```python
from build123d import *

# Parameters (mm, degrees)
F1_DEPTH = 100
F2_T     = -12
F4_W     = 187.6861900091
F4_H     = 13.1353894249
F5_DEPTH = 200


with BuildPart() as f1:
    # F0 (on Right) → F1 (new body, symmetric)
    with BuildSketch(Plane.YZ):
        Polygon((-193.7253567732, -86.0714143496), (-193.7253567732, -126.0714143496), (156.2746432268, -126.0714143496), (156.2746432268, 123.9285856504), (76.2746432268, 123.9285856504), align=None)
    extrude(amount=F1_DEPTH, both=True)

    # F2
    f2_openings = [f1.faces().sort_by_distance(p)[0] for p in [
        (0, -58.725357, 18.928586),
    ]]
    offset(amount=F2_T, openings=f2_openings)

    # F4 (on face) → F5 (join)
    with BuildSketch(Plane.YZ.offset(100)):
        with Locations((59.6075579524, 6.5676947124)):
            Rectangle(F4_W, F4_H)
    extrude(amount=-F5_DEPTH)


solid = f1.part
```
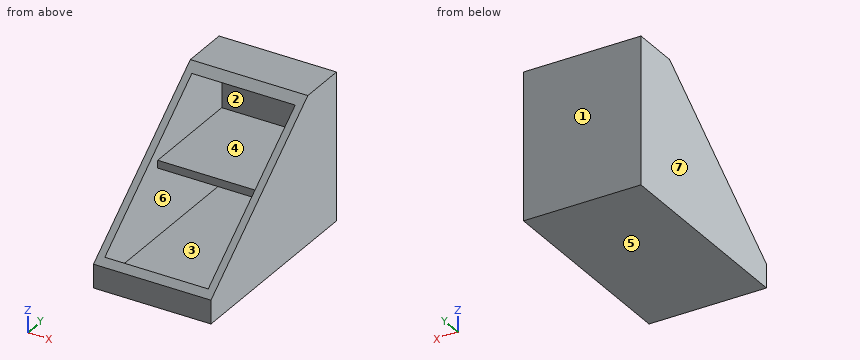
Work out the finished part from the listing and answer in its coordinate system (mm). Face numbers are marked on the shaded views. A direction names the side the tool comes from. Give positions to 0.01 mm unless a question says otherwise; leave off trailing zeros. Loops run counter-clockwise (first coordinate to the right, second up) from the corner with the lowest first, then second, coordinate; pieces in that order, holes last. Notation, with made-up numbers: (-24, 55.25) - (20, 55.25) arc R23 cw to (20, 86.25) - close; hole circle Ø2 at (-2, 78.25). An arc over 180 degrees is marked (long way). Use CSV: the item, a comma, the result in double quotes. Start each with the question number.
(1) Determine the mould class of the marked faces 4, 5, 6 and 7 for opening direction Z: released by +Z, released by -Z, zero draft, split by the parting line, or undercut.
(2) Find section C-C, the plane z = -61. Determine the outline of the cut face in (x, y), plus the area to 3 significant figures.
(3) Find section B-B, the plane x = 29. Determine the outline of the cut face in (y, z), plus the area to 3 significant figures.
(4) Each of these flat-tipped pins is pushed along its axis until it touches: pin 1 (3 mm diameter, centred on x = -21, z = -83.5, fed in from -Y); pin 2 (8 mm diameter, centred on x = 37.5, z = 17, fed in from -Y). Where does it stop, or does it pass through?
(5) Find section D-D, the plane y = -2. Determine the outline of the cut face in (x, z), plus the area to 3 significant figures.
(6) A tool of negligible diameter and unlimited length cuts with its end or side. For the marked faces 1, 2 and 3, from which of +Z, -Z, +X, -X, +Y, -Y can it reach the whole face along a straight path? Write none if from no direction.
(7) Find the intervals of material crossed by L1, parallel to Z at x = 69, y = 84.5; L2, parallel to X at y = 87, z = 15.5; L3, parallel to Y at x = -36, z = -103, in increasing order.
(8) Find section A-A, the plane y = 108.5. Determine the outline of the cut face in (x, z), plus the area to 3 significant figures.
Results found:
1,face 4,"undercut"
1,face 5,"released by -Z"
1,face 6,"undercut"
1,face 7,"zero draft"
2,outline,"(-100, -161.49) - (-88, -161.49) - (-88, 144.27) - (88, 144.27) - (88, -161.49) - (100, -161.49) - (100, 156.27) - (-100, 156.27) - close"
2,area,"9,740 mm^2"
3,outline,"(-193.73, -126.07) - (156.27, -126.07) - (156.27, 123.93) - (76.27, 123.93) - (60.85, 111.93) - (144.27, 111.93) - (144.27, 13.14) - (-34.24, 13.14) - (-34.24, 0) - (144.27, 0) - (144.27, -114.07) - (-181.73, -114.07) - (-181.73, -76.74) - (-193.73, -86.07) - close"
3,area,"10,700 mm^2"
4,pin 1,"y = -192.35"
4,pin 2,"y = -34.24"
5,outline,"(-100, -126.07) - (100, -126.07) - (100, 63.05) - (88, 63.05) - (88, 13.14) - (-88, 13.14) - (-88, 63.05) - (-100, 63.05) - close; hole (-88, -114.07) - (88, -114.07) - (88, 0) - (-88, 0) - close"
5,area,"8,960 mm^2"
6,face 1,"+Z, -Z, +X, -X, +Y"
6,face 2,"-Y"
6,face 3,"none"
7,L1,"-126.07 to -114.07, 0 to 13.14, 111.93 to 123.93"
7,L2,"-100 to -88, 88 to 100"
7,L3,"-193.73 to -181.73, 144.27 to 156.27"
8,outline,"(-100, -126.07) - (100, -126.07) - (100, 123.93) - (-100, 123.93) - close; hole (-88, -114.07) - (88, -114.07) - (88, 0) - (-88, 0) - close; hole (-88, 13.14) - (88, 13.14) - (88, 111.93) - (-88, 111.93) - close"
8,area,"12,500 mm^2"
